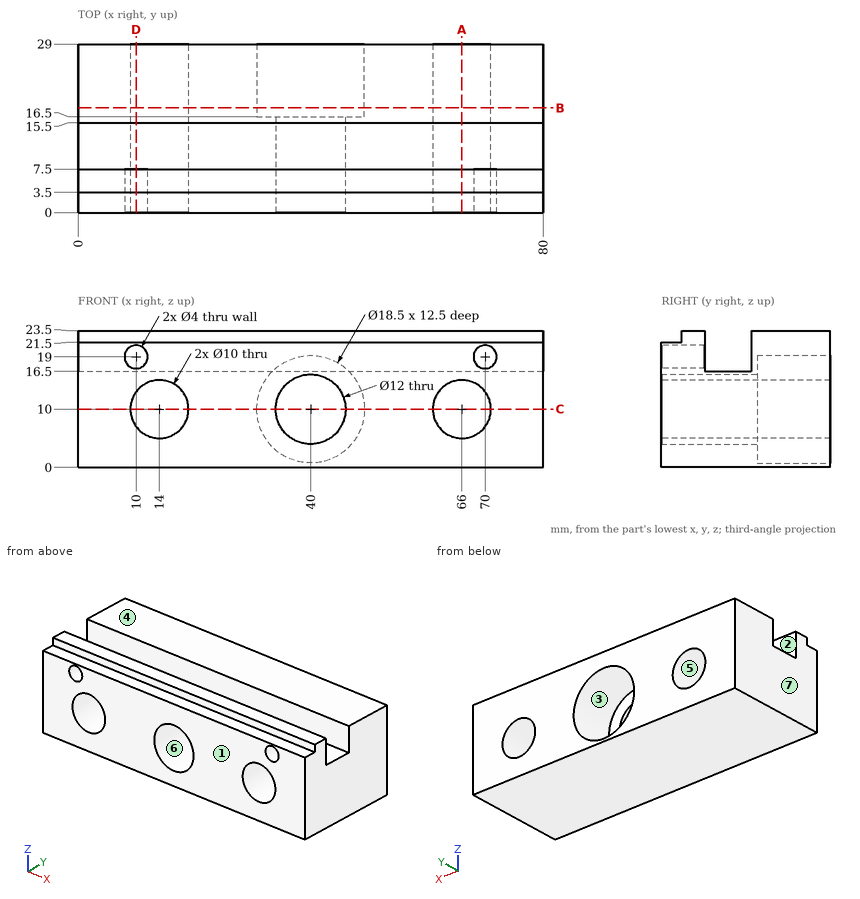
Here's the drawing with two shaded views (mm, measured from the low corner). I have some questions. A direction names the side the tool comes from. Give positions to 0.01 mm unless a question says otherwise; leave off trailing zeros. Loops run counter-clockwise (first coordinate to the right, second up) from the corner with the lowest first, then second, coordinate; pieces in that order, holes last. Notation, with made-up numbers: (62.25, 6) - (98.25, 6) arc R36 cw to (98.25, 42) - close; hole circle Ø7 at (17, -15.5). An arc over 180 degrees is marked (long way). One line per item, written item: value.
(1) If we section it at A-A, the plane x = 66: List the corners of the cut face in (y, z) for me.
Verdict:
outline: (0, 0) - (29, 0) - (29, 5) - (0, 5) - close; (0, 15) - (29, 15) - (29, 23.5) - (15.5, 23.5) - (15.5, 16.5) - (7.5, 16.5) - (7.5, 23.5) - (3.5, 23.5) - (3.5, 21.5) - (0, 21.5) - close
(2) I'm going to push flat-ended pins straight in: pin 1 (6 mm diameter, centred on x = 14, z = 10, fed in from -Y); pin 2 (9 mm diameter, centred on x = 42, z = 12.5, fed in from +Y); pin 3 (0.6 mm diameter, centred on x = 59.5, z = 22.5, fed in from -Y). Where does each tip first touch, or does it pass through?
Verdict:
pin 1: through
pin 2: y = 16.5
pin 3: y = 3.5
(3) If we section it at D-D, the plane x = 10: List the corners of the cut face in (y, z) for me.
Verdict:
outline: (0, 0) - (29, 0) - (29, 7) - (0, 7) - close; (0, 13) - (29, 13) - (29, 23.5) - (15.5, 23.5) - (15.5, 16.5) - (7.5, 16.5) - (7.5, 17) - (0, 17) - close; (0, 21) - (7.5, 21) - (7.5, 23.5) - (3.5, 23.5) - (3.5, 21.5) - (0, 21.5) - close
(4) On a 3-axis mill with a long thin cutter (end or side, diameter ignored), from which of +Z, -Z, +X, -X, +Y, -Y can I reach the whole of each face in a straight line? I mean the marked faces 1, 2 and 3. Say none if no direction works.
Verdict:
face 1: +Z, -Z, +X, -X, -Y
face 2: +Z, +X, -X
face 3: +Y
(5) If we mould it in two halves opening along Z, with no side actions, what happens to the marked faces 4, 5, 6 and 7? For each: released by +Z, released by -Z, zero draft, split by the parting line, or undercut.
Verdict:
face 4: released by +Z
face 5: undercut
face 6: undercut
face 7: zero draft
(6) If we section it at B-B, the plane y = 18: List the corners of the cut face in (x, z) for me.
Verdict:
outline: (0, 0) - (80, 0) - (80, 23.5) - (0, 23.5) - close; hole circle Ø10 at (14, 10); hole circle Ø18.5 at (40, 10); hole circle Ø10 at (66, 10)
(7) If we section it at C-C, the plane z = 10: List the corners of the cut face in (x, y) for me, plus the area to 3 significant figures.
Verdict:
outline: (0, 0) - (9, 0) - (9, 29) - (0, 29) - close; (19, 0) - (34, 0) - (34, 16.5) - (30.75, 16.5) - (30.75, 29) - (19, 29) - close; (46, 0) - (61, 0) - (61, 29) - (49.25, 29) - (49.25, 16.5) - (46, 16.5) - close; (71, 0) - (80, 0) - (80, 29) - (71, 29) - close
area: 1,310 mm^2
(8) I need wall thicknesses on line 1 along Y through (x, z) = (12, 22); line 2 along Y through (x, z) = (46.5, 18.75); line 3 along Z through (x, y) = (66, 22.5). Which ranges of each line are inside material? Lowest first, please.
Verdict:
line 1: 3.5 to 7.5, 15.5 to 29
line 2: 0 to 7.5, 15.5 to 29
line 3: 0 to 5, 15 to 23.5
